Design review of the part built by this model. Coordinates are the model's own, in mm. A direction names the side the tool comes from. Round coordinates to 2 decimals unless told otherwise and drop trailing zeros. Order: outer loops, then holes, each group sorted by start corner. A loop starts at its lowest first (then second) coordinate and runs counter-clockwise, first axis right, second up. Notation, with made-up numbers: (8, 84) - (34, 84) arc R20 cw to (34, 108) - close; hole circle Ø2 at (3.25, -18). An arc over 180 degrees is marked (long way). Write item = value, one per line.
from build123d import *

# Parameters (mm, degrees)
SKETCH1_W           = 140
SKETCH1_H           = 90
BOSS_EXTRUDE1_DEPTH = 2
SKETCH2_W           = 10
SKETCH2_H           = 10
BOSS_EXTRUDE2_DEPTH = 50
CHAMFER1_SIZE       = 5
SKETCH3_R           = 1.5
CUT_EXTRUDE1_DEPTH  = 53
SKETCH4_R           = 1.5
CUT_EXTRUDE2_DEPTH  = 3
CUT_EXTRUDE3_DEPTH  = 3


with BuildPart() as part:
    # Sketch1 → Boss-Extrude1 (new body)
    with BuildSketch(Plane(origin=(0, 0, 0), x_dir=(1, 0, 0), z_dir=(0, 1, 0))):
        Rectangle(SKETCH1_W, SKETCH1_H)
    extrude(amount=BOSS_EXTRUDE1_DEPTH)

    # Sketch2 → Boss-Extrude2 (add)
    with BuildSketch(Plane(origin=(0, 2, 0), x_dir=(1, 0, 0), z_dir=(0, 1, 0))):
        with Locations((-65, 40)):
            Rectangle(SKETCH2_W, SKETCH2_H)
        with Locations((65, 40)):
            Rectangle(SKETCH2_W, SKETCH2_H)
        with Locations((65, -40)):
            Rectangle(SKETCH2_W, SKETCH2_H)
        with Locations((-65, -40)):
            Rectangle(SKETCH2_W, SKETCH2_H)
    extrude(amount=BOSS_EXTRUDE2_DEPTH)

    # Chamfer1
    chamfer1_edges = [part.edges().sort_by_distance(p)[0] for p in [
        (-65, 2, -35),
        (-60, 2, -40),
        (60, 2, -40),
        (65, 2, -35),
        (65, 2, 35),
        (60, 2, 40),
        (-60, 2, 40),
        (-65, 2, 35),
    ]]
    chamfer(chamfer1_edges, length=CHAMFER1_SIZE)

    # Sketch3 → Cut-Extrude1 (cut, through all)
    with BuildSketch(Plane(origin=(0, 52, 0), x_dir=(1, 0, 0), z_dir=(0, 1, 0))):
        with Locations((-65, 40)):
            Circle(SKETCH3_R)
        with Locations((65, 40)):
            Circle(SKETCH3_R)
        with Locations((65, -40)):
            Circle(SKETCH3_R)
        with Locations((-65, -40)):
            Circle(SKETCH3_R)
    extrude(amount=-CUT_EXTRUDE1_DEPTH, mode=Mode.SUBTRACT)

    # Sketch4 → Cut-Extrude2 (cut, through all)
    with BuildSketch(Plane(origin=(0, 2, 0), x_dir=(1, 0, 0), z_dir=(0, 1, 0))):
        with Locations((-40, 0)):
            Circle(SKETCH4_R)
        with Locations((10, 0)):
            Circle(SKETCH4_R)
    extrude(amount=-CUT_EXTRUDE2_DEPTH, mode=Mode.SUBTRACT)

    # Sketch5 → Cut-Extrude3 (cut, through all)
    with BuildSketch(Plane(origin=(0, 2, 0), x_dir=(1, 0, 0), z_dir=(0, 1, 0))):
        with BuildLine():
            Line((24, 35.63), (36, 35.63))
            ThreePointArc((36, 35.63), (38.25, 33.38), (36, 31.13))
            Line((36, 31.13), (24, 31.13))
            ThreePointArc((24, 31.13), (21.75, 33.38), (24, 35.63))
        make_face()
    cut_extrude3 = extrude(amount=-CUT_EXTRUDE3_DEPTH, mode=Mode.SUBTRACT)

    # Mirror1: Cut-Extrude3 across plane
    add(cut_extrude3.mirror(Plane.XY), mode=Mode.SUBTRACT)


solid = part.part
1) To check wall thickness, follow L1, parallel to Z at x = 65, y = 18; L2, parallel to X at y = 32.5, z = 40; L3, parallel to Y at x = 46, z = 1. State the ranges of each line that lie inside material, in increasing order. Write a range as from..to.
Findings:
L1 = -45..-41.5, -38.5..-35, 35..38.5, 41.5..45
L2 = -70..-66.5, -63.5..-60, 60..63.5, 66.5..70
L3 = 0..2
2) Clearance check with flat-ended pins moving along their axes: pin 1 Ø2.5 at (x, z) = (-65, 40) entering from +Y; pin 2 Ø1.5 at (x, z) = (-17, 9.5) entering from -Y; pin 3 Ø3.5 at (x, z) = (10, 0) entering from +Y. State where each tip first meets the part, or that it passes through.
Findings:
pin_1 = through
pin_2 = 0
pin_3 = 2
3) We need section A-A on x = 10. Write out the cut boundary in (y, z).
Findings:
outline = (0, -45) - (2, -45) - (2, -1.5) - (0, -1.5) - close; (0, 1.5) - (2, 1.5) - (2, 45) - (0, 45) - close
4) The part is to be moulded in two halves that separate along X. For faces 1 (the flat face through (63.8, 52, -41.2)), 2 (the flat face through (-58, 5, 39)), 3 (the cylindrical face through (-41.5, 1.01, -0.07)), say which applies: released by +X, released by -X, zero draft, split by the parting line, or undercut.
Findings:
face_1 = zero draft
face_2 = undercut
face_3 = undercut
5) We need section C-C on y = 20.5. Write out the cut boundary in (x, z).
Findings:
outline = (-70, -45) - (-60, -45) - (-60, -35) - (-70, -35) - close; (-70, 35) - (-60, 35) - (-60, 45) - (-70, 45) - close; (60, -45) - (70, -45) - (70, -35) - (60, -35) - close; (60, 35) - (70, 35) - (70, 45) - (60, 45) - close; hole circle Ø3 at (-65, -40); hole circle Ø3 at (-65, 40); hole circle Ø3 at (65, -40); hole circle Ø3 at (65, 40)
6) We need section B-B on z = -40. Write out the cut boundary in (x, y), and give its area (3 significant figures).
Findings:
outline = (-70, 0) - (-66.5, 0) - (-66.5, 52) - (-70, 52) - close; (-63.5, 0) - (63.5, 0) - (63.5, 52) - (60, 52) - (60, 7) - (55, 2) - (-55, 2) - (-60, 7) - (-60, 52) - (-63.5, 52) - close; (66.5, 0) - (70, 0) - (70, 52) - (66.5, 52) - close
area = 993 mm^2
7) For faces 4 (the flat face through (60, 29, -40)), 5 (the flat face through (65, 29, -35)), 6 (the cylindrical face through (8.5, 1.01, -0.07)), list the 3-axis set-ups (+Z, -Z, +X, -X, +Y, -Y) from which the entire face can be reached by the end or side of a thin tool; tool diameter is ignored.
Findings:
face_4 = +Z, -Z, +Y
face_5 = +X, -X, +Y
face_6 = +Y, -Y
8) We need section D-D on x = 65. Write out the cut boundary in (y, z).
Findings:
outline = (0, -45) - (52, -45) - (52, -41.5) - (0, -41.5) - close; (0, -38.5) - (52, -38.5) - (52, -35) - (7, -35) - (2, -30) - (2, 30) - (7, 35) - (52, 35) - (52, 38.5) - (0, 38.5) - close; (0, 41.5) - (52, 41.5) - (52, 45) - (0, 45) - close
